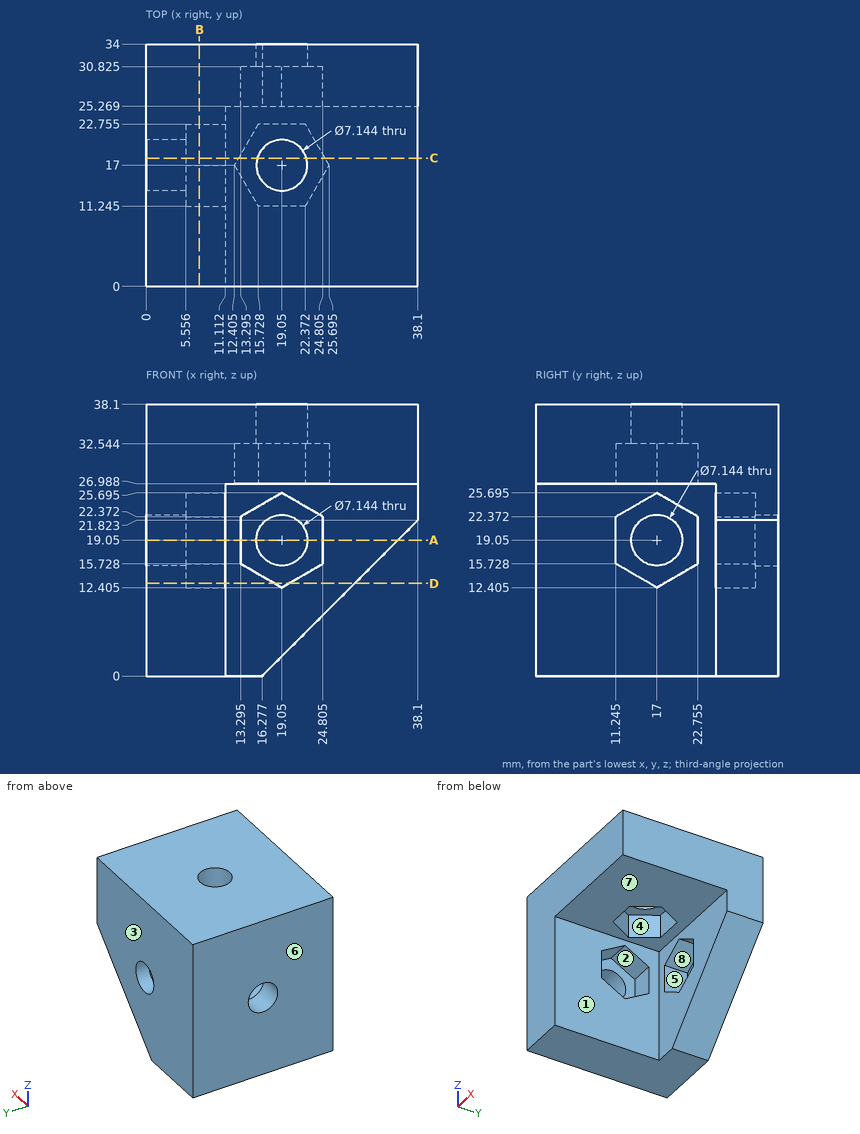
Drawing for the job (mm, zero at the part's lowest x, y, z). A direction names the side the tool comes from. Coordinates: 2 decimals unless noted, no trailing zeros. Loops run counter-clockwise (first coordinate to the right, second up) from the corner with the lowest first, then second, coordinate; pieces in that order, holes last. Notation, with made-up numbers: (12, 11) - (21, 11) arc R25 ccw to (21, 44) - close; hole circle Ø3 at (11, 38). An arc over 180 degrees is marked (long way). Return JSON: item names as keys, results as strings.
1. Probe L1, parallel to Y at x = 28, z = 15; L2, parallel to Y at x = 19, z = 35; L3, parallel to X at y = 32, z = 9 (1 decimal). List the from-to ranges inside material, lowest first. Write a range as from..to.
Result:
{"L1": "y = 25.27..34", "L2": "y = 0..13.43, 20.57..34", "L3": "x = 0..25.3"}
2. Band-saw the part on B-B (x = 7.5). Give the cut face in (y, z) (1 decimal).
Result:
{"outline": "(0, 0) - (34, 0) - (34, 38.1) - (0, 38.1) - close; hole (11.2, 15.7) - (17, 12.4) - (22.8, 15.7) - (22.8, 22.4) - (17, 25.7) - (11.2, 22.4) - close"}
3. 3-axis set-ups, long thin cutter, end or side, ignore diameter. For the marked faces 1, 2, 3, 4 and 5: which of +Z, -Z, +X, -X, +Y, -Y reach the whole face in a straight line?
Result:
{"face 1": "-Z, +X, -Y", "face 2": "+X", "face 3": "+Z, -Z, +X, -X, +Y", "face 4": "-Z", "face 5": "-Y"}
4. Band-saw the part on A-A (z = 19.05). Give the cut face in (x, y) (1 decimal).
Result:
{"outline": "(0, 0) - (11.1, 0) - (11.1, 11.2) - (5.6, 11.2) - (5.6, 13.4) - (0, 13.4) - close; (0, 20.6) - (5.6, 20.6) - (5.6, 22.8) - (11.1, 22.8) - (11.1, 25.3) - (13.3, 25.3) - (13.3, 30.8) - (15.5, 30.8) - (15.5, 34) - (0, 34) - close; (22.6, 30.8) - (24.8, 30.8) - (24.8, 25.3) - (35.3, 25.3) - (35.3, 34) - (22.6, 34) - close"}
5. Band-saw the part on D-D (z = 13). Give the cut face in (x, y) (1 decimal).
Result:
{"outline": "(0, 0) - (11.1, 0) - (11.1, 16) - (5.6, 16) - (5.6, 18) - (11.1, 18) - (11.1, 25.3) - (18, 25.3) - (18, 30.8) - (20.1, 30.8) - (20.1, 25.3) - (29.3, 25.3) - (29.3, 34) - (0, 34) - close"}
6. Band-saw the part on C-C (y = 18). Give the cut face in (x, z).
Result:
{"outline": "(0, 0) - (11.11, 0) - (11.11, 12.98) - (5.56, 12.98) - (5.56, 15.62) - (0, 15.62) - close; (0, 22.48) - (5.56, 22.48) - (5.56, 25.12) - (11.11, 25.12) - (11.11, 26.99) - (12.98, 26.99) - (12.98, 32.54) - (15.62, 32.54) - (15.62, 38.1) - (0, 38.1) - close; (22.48, 32.54) - (25.12, 32.54) - (25.12, 26.99) - (38.1, 26.99) - (38.1, 38.1) - (22.48, 38.1) - close"}
7. Drop flat-ended pins along their axis: pin 1 (1 mm diameter, centred on y = 13.5, z = 25.5, fed in from +X); pin 2 (6 mm diameter, centred on y = 27, z = 21, fed in from +X); pin 3 (7.5 mm diameter, centred on x = 25, y = 11.5, fed in from -Z); pin 4 (9 mm diameter, centred on x = 18.5, z = 21, fed in from -Y). Give the stop position or say it passes through.
Result:
{"pin 1": "stops at x = 11.11", "pin 2": "stops at x = 38.1", "pin 3": "stops at z = 26.99", "pin 4": "stops at y = 25.27"}
8. Mould opens along Z. For the marked faces 6, 7 and 8 say: released by +Z, released by -Z, zero draft, split by the parting line, or undercut.
Result:
{"face 6": "zero draft", "face 7": "released by -Z", "face 8": "undercut"}
